Source: CAD feature listing. Evaluate the final solid. Frame: model axes, mm. Face numbers are marked on the shaded views. A direction names the side the tool comes from. Round coordinates to 2 decimals unless told otherwise and drop trailing zeros. Loops run counter-clockwise (first coordinate to the right, second up) from the corner with the lowest first, then second, coordinate; pieces in that order, holes last. Notation, with made-up numbers: M -21,-11.75 L 20,-11.75 A28 ccw 20,26.25 Z; hole C 29,-27 d6. An arc over 180 degrees is marked long. Answer as CSV lines item,"result". Start each with the question number.
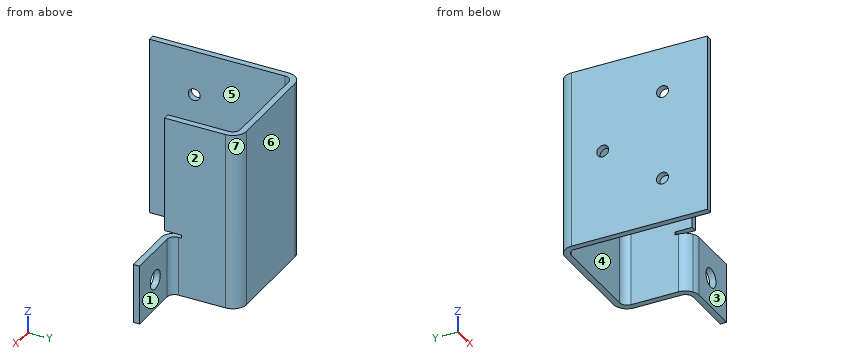
```python
from build123d import *

# Parameters (mm, degrees)
BASE_FLANGE1_DEPTH    = 76.2
SKETCH5_R             = 2.54
CUT_EXTRUDE1_DEPTH    = 111.256309818
MITER_FLANGE1_DEPTH   = 26.72842
MITER_START           = 25.4
MITER_FLANGE1_2_DEPTH = 1.32842
MITER_FLANGE1_3_DEPTH = 25.4
SKETCH7_R             = 4.056943783
CUT_EXTRUDE2_DEPTH    = 114.122546996


# Read off the part's stored shape, not the designer's step: Miter Flange1
# Sheet-metal steps are written as plain solids
with BuildPart() as part:
    # Sketch3 → Base-Flange1 (new body)
    with BuildSketch(Plane.XY):
        with BuildLine():
            Line((50.8, 31.75), (50.8, 57.66816))
            ThreePointArc((50.8, 57.66816), (49.091893611, 61.791893611), (44.96816, 63.5))
            Line((44.96816, 63.5), (5.83184, 63.5))
            ThreePointArc((5.83184, 63.5), (1.708106389, 61.791893611), (0, 57.66816))
            Line((0, 57.66816), (0, 0))
            Line((0, 0), (2.65684, 0))
            Line((2.65684, 0), (2.65684, 57.66816))
            ThreePointArc((2.65684, 57.66816), (3.58677597, 59.91322403), (5.83184, 60.84316))
            Line((5.83184, 60.84316), (44.96816, 60.84316))
            ThreePointArc((44.96816, 60.84316), (47.21322403, 59.91322403), (48.14316, 57.66816))
            Line((48.14316, 57.66816), (48.14316, 31.75))
            Line((48.14316, 31.75), (50.8, 31.75))
        make_face()
    extrude(amount=BASE_FLANGE1_DEPTH)

    # Sketch5 → Cut-Extrude1 (cut, through all)
    with BuildSketch(Plane(origin=(2.65684, 0, 0), x_dir=(0, 0, -1), z_dir=(1, 0, 0))):
        with Locations(Location((-57.15, 19.05, 0), (0, 0, 90))):
            Circle(SKETCH5_R)
        with Locations(Location((-38.1, 44.45, 0), (0, 0, 90))):
            Circle(SKETCH5_R)
        with Locations(Location((-19.05, 19.05, 0), (0, 0, 90))):
            Circle(SKETCH5_R)
    extrude(amount=-CUT_EXTRUDE1_DEPTH, mode=Mode.SUBTRACT)

    # Miter Flange1 outline → Miter Flange1 (cut)
    with BuildSketch(Plane.XY):
        with BuildLine():
            Line((50.8, 31.75), (50.8, 32.690037389))
            ThreePointArc((50.8, 32.690037389), (48.850234162, 34.798472814), (48.14316, 37.58184))
            Line((48.14316, 37.58184), (48.14316, 31.75))
            Line((48.14316, 31.75), (50.8, 31.75))
        make_face()
    extrude(amount=MITER_FLANGE1_DEPTH, mode=Mode.SUBTRACT)

    # Miter Flange1 2 outline → Miter Flange1 2 (cut)
    with BuildSketch(Plane.XY.offset(MITER_START)):
        with BuildLine():
            ThreePointArc((48.14316, 37.58184), (48.850234162, 34.798472814), (50.8, 32.690037389))
            Line((50.8, 32.690037389), (50.8, 38.91026))
            Line((50.8, 38.91026), (48.14316, 38.91026))
            Line((48.14316, 38.91026), (48.14316, 37.58184))
        make_face()
    extrude(amount=MITER_FLANGE1_2_DEPTH, mode=Mode.SUBTRACT)

    # Miter Flange1 3 outline → Miter Flange1 3 (add)
    with BuildSketch(Plane.XY):
        with BuildLine():
            Line((53.975, 31.75), (76.2, 31.75))
            Line((76.2, 31.75), (76.2, 34.40684))
            Line((76.2, 34.40684), (53.975, 34.40684))
            ThreePointArc((53.975, 34.40684), (51.72993597, 35.33677597), (50.8, 37.58184))
            Line((50.8, 37.58184), (50.8, 32.690037389))
            ThreePointArc((50.8, 32.690037389), (52.319381136, 31.989945512), (53.975, 31.75))
        make_face()
    extrude(amount=MITER_FLANGE1_3_DEPTH)

    # Sketch7 → Cut-Extrude2 (cut, through all)
    with BuildSketch(Plane(origin=(0, 34.40684, 0), x_dir=(-1, 0, 0), z_dir=(0, 1, 0))):
        with Locations((-63.5, 12.7)):
            Circle(SKETCH7_R)
    extrude(amount=-CUT_EXTRUDE2_DEPTH, mode=Mode.SUBTRACT)


solid = part.part
```
1) Access query for the marked faces 1, 2, 3 and 4. Directions: +Z, -Z, +X, -X, +Y, -Y. A direction counts if a zero-diameter tool reaches every point of the face in a straight line with its end or side. Return the directions, or none.
2) Section D-D, the plane y = 44.45. Return loops of the section in (x, z).
3) Ray query, line 1 along Z through (x, y) = (0.8, 19.05); line 2 along Z through (x, y) = (0.6, 44.45); line 3 along X through (y, z) = (52, 34). Return the intervals inside material, ascending.
4) Contact query for flat-ended pins moving along their axis: pin 1 Ø8 at (y, z) = (42.5, 31.5) entering from +X; pin 2 Ø2 at (x, z) = (49.5, 61) entering from -Y; pin 3 Ø6.5 at (x, z) = (62, 18) entering from +Y. Output: stop coordinate, or through.
5) Section B-B, the plane y = 19.05. Return loops of the section in (x, z), and give its area (3 significant figures).
6) Section A-A, the plane z = 19.05. Return loops of the section in (x, y) (3 decimals).
7) Section C-C, the plane z = 38.1. Return loops of the section in (x, y) (3 decimals), and give its area (3 significant figures).
8) Mould query, pull axis X, two halves, no side actions, for the marked faces 5, 6 and 7. Classes: pulls with the +X half, pulls with the -X half, needs draft (parallel to the pull), parting line crosses it, or undercut.
Findings below:
1,face 1,"+Z, -Z, +X, +Y"
1,face 2,"+Z, +X, +Y"
1,face 3,"+Z, -Z, +X, -Y"
1,face 4,"+Z, -Z, -Y"
2,outline,"M 0,0 L 2.66,0 L 2.66,35.56 L 0,35.56 Z; M 0,40.64 L 2.66,40.64 L 2.66,76.2 L 0,76.2 Z; M 48.14,0 L 50.8,0 L 50.8,76.2 L 48.14,76.2 Z"
3,line 1,"0 to 16.51, 21.59 to 54.61, 59.69 to 76.2"
3,line 2,"0 to 35.56, 40.64 to 76.2"
3,line 3,"0 to 2.66, 48.14 to 50.8"
4,pin 1,"x = 50.8"
4,pin 2,"y = 31.75"
4,pin 3,"y = 34.41"
5,outline,"M 0,0 L 2.66,0 L 2.66,16.51 L 0,16.51 Z; M 0,21.59 L 2.66,21.59 L 2.66,54.61 L 0,54.61 Z; M 0,59.69 L 2.66,59.69 L 2.66,76.2 L 0,76.2 Z"
5,area,"175 mm²"
6,outline,"M 0,0 L 2.657,0 L 2.657,16.51 L 0,16.51 Z; M 0,21.59 L 2.657,21.59 L 2.657,57.668 A3.175 cw 5.832,60.843 L 44.968,60.843 A3.175 cw 48.143,57.668 L 48.143,37.582 A5.832 ccw 53.975,31.75 L 76.2,31.75 L 76.2,34.407 L 53.975,34.407 A3.175 cw 50.8,37.582 L 50.8,57.668 A5.832 ccw 44.968,63.5 L 5.832,63.5 A5.832 ccw 0,57.668 Z"
7,outline,"M 0,0 L 2.657,0 L 2.657,41.91 L 0,41.91 Z; M 0,46.99 L 2.657,46.99 L 2.657,57.668 A3.175 cw 5.832,60.843 L 44.968,60.843 A3.175 cw 48.143,57.668 L 48.143,31.75 L 50.8,31.75 L 50.8,57.668 A5.832 ccw 44.968,63.5 L 5.832,63.5 A5.832 ccw 0,57.668 Z"
7,area,"350 mm²"
8,face 5,"undercut"
8,face 6,"needs draft"
8,face 7,"pulls with the +X half"
